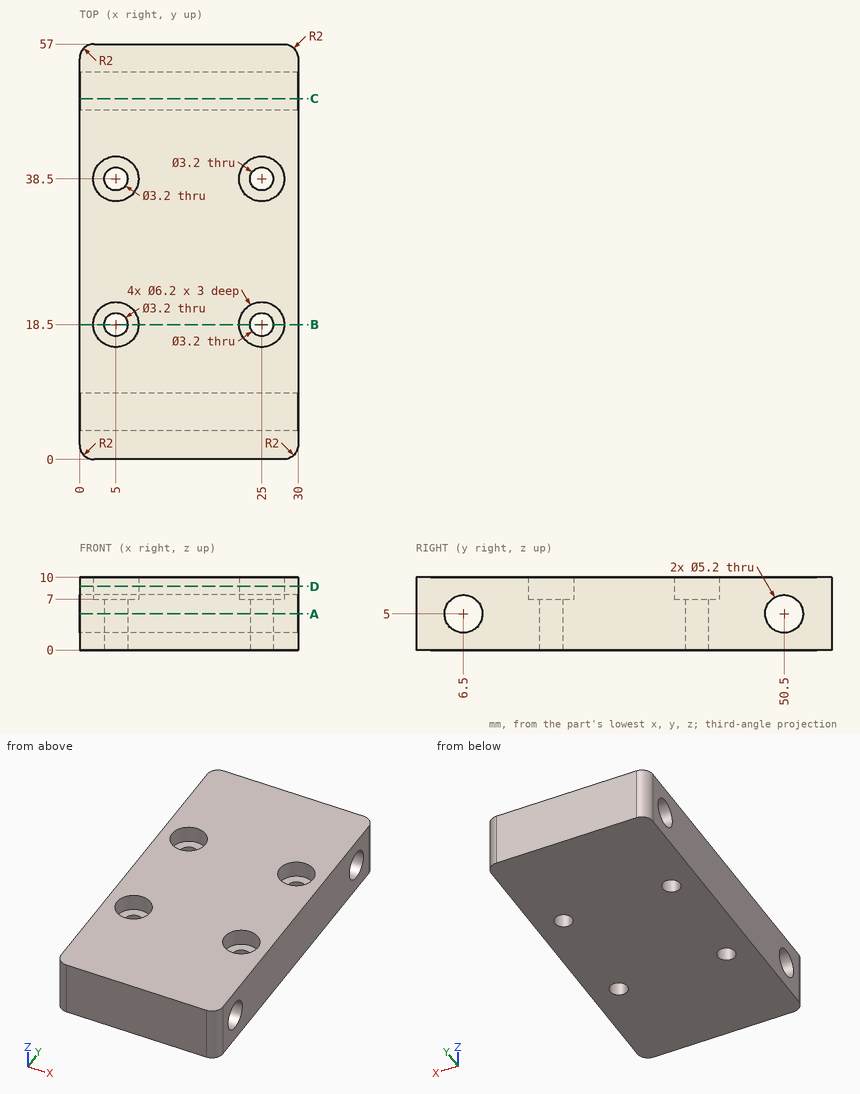
Drawing for the job (mm, zero at the part's lowest x, y, z). Round coordinates to 2 decimals unless told otherwise and drop trailing zeros. Loops run counter-clockwise (first coordinate to the right, second up) from the corner with the lowest first, then second, coordinate; pieces in that order, holes last. Notation, with made-up numbers: (-14, -12.75) - (-8, -12.75) arc R6 cw to (-8, -7.75) - close; hole circle Ø10 at (-35, -25.5). An arc over 180 degrees is marked (long way). Return JSON: item names as keys, results as strings. Group by question number.
Q1. Band-saw the part on A-A on z = 5. Give the cut face in (x, y), plus the area to 3 significant figures.
Q2. Flat gauge pins, fed straight in: pin 1 Ø4 at (x, z) = (19, 2) entering from -Y; pin 2 Ø3.5 at (x, y) = (5, 18.5) entering from +Z. Where does each tip first touch, or does it go through?
Q3. Band-saw the part on B-B on y = 18.5. Give the cut face in (x, z), plus the area to 3 significant figures.
Q4. Band-saw the part on C-C on y = 49.5. Give the cut face in (x, z).
Q5. Band-saw the part on D-D on z = 8.75. Give the cut face in (x, y), plus the area to 3 significant figures.
Q6. Drill centre lines: line 1 along X through (y, z) = (38.5, 4.5); line 2 along X through (y, z) = (18.5, 9.25); line 3 along Y through (x, z) = (5, 4.75). Where is each one in solid material? Low to high. Write a range as [from, to].
Solutions:
{
 "1": {"outline": "(0, 2) arc R2 ccw to (2, 0) - (28, 0) arc R2 ccw to (30, 2) - (30, 3.9) - (0, 3.9) - close; (0, 9.1) - (30, 9.1) - (30, 47.9) - (0, 47.9) - close; (0, 53.1) - (30, 53.1) - (30, 55) arc R2 ccw to (28, 57) - (2, 57) arc R2 ccw to (0, 55) - close; hole circle Ø3.2 at (5, 18.5); hole circle Ø3.2 at (5, 38.5); hole circle Ø3.2 at (25, 18.5); hole circle Ø3.2 at (25, 38.5)", "area": "1,360 mm^2"},
 "2": {"pin 1": "stops at y = 0", "pin 2": "stops at z = 7"},
 "3": {"outline": "(0, 0) - (3.4, 0) - (3.4, 7) - (1.9, 7) - (1.9, 10) - (0, 10) - close; (6.6, 0) - (23.4, 0) - (23.4, 7) - (21.9, 7) - (21.9, 10) - (8.1, 10) - (8.1, 7) - (6.6, 7) - close; (26.6, 0) - (30, 0) - (30, 10) - (28.1, 10) - (28.1, 7) - (26.6, 7) - close", "area": "218 mm^2"},
 "4": {"outline": "(0, 0) - (30, 0) - (30, 2.6) - (0, 2.6) - close; (0, 7.4) - (30, 7.4) - (30, 10) - (0, 10) - close"},
 "5": {"outline": "(0, 2) arc R2 ccw to (2, 0) - (28, 0) arc R2 ccw to (30, 2) - (30, 55) arc R2 ccw to (28, 57) - (2, 57) arc R2 ccw to (0, 55) - close; hole circle Ø6.2 at (5, 18.5); hole circle Ø6.2 at (5, 38.5); hole circle Ø6.2 at (25, 18.5); hole circle Ø6.2 at (25, 38.5)", "area": "1,590 mm^2"},
 "6": {"line 1": "x = [0, 3.4], [6.6, 23.4], [26.6, 30]", "line 2": "x = [0, 1.9], [8.1, 21.9], [28.1, 30]", "line 3": "y = [0, 3.91], [9.09, 16.9], [20.1, 36.9], [40.1, 47.91], [53.09, 57]"}
}
